from build123d import *

# Parameters (mm, degrees)
BASE_FLANGE1_DEPTH   = 12.5
M4_CLEARANCE_HOLE1_D = 4.5


# Sheet-metal steps are written as plain solids
with BuildPart() as part:
    # Sketch1 → Base-Flange1 (new, symmetric)
    with BuildSketch(Plane(origin=(0, 0, 0), x_dir=(1, 0, 0), z_dir=(0, 1, 0))):
        with BuildLine():
            Line((0, 0), (-12, 0))
            ThreePointArc((-12, 0), (-14.121320344, 0.878679656), (-15, 3))
            Line((-15, 3), (-15, 98.5))
            ThreePointArc((-15, 98.5), (-15.439339828, 99.560660172), (-16.5, 100))
            Line((-16.5, 100), (-95, 100))
            Line((-95, 100), (-95, 101.5))
            Line((-95, 101.5), (-16.5, 101.5))
            ThreePointArc((-16.5, 101.5), (-14.378679656, 100.621320344), (-13.5, 98.5))
            Line((-13.5, 98.5), (-13.5, 3))
            ThreePointArc((-13.5, 3), (-13.060660172, 1.939339828), (-12, 1.5))
            Line((-12, 1.5), (0, 1.5))
            Line((0, 1.5), (0, 0))
        make_face()
    extrude(amount=BASE_FLANGE1_DEPTH, both=True)

    # M4 Clearance Hole1 (through all)
    with Locations(Plane.XY):
        with Locations((-4, 7), (-4, -7)):
            Hole(M4_CLEARANCE_HOLE1_D / 2)


solid = part.part
For this review, take the finished solid that the model builds, in its own axes (mm). A direction names the side the tool comes from. Coordinates: 2 decimals unless noted, no trailing zeros. Loops run counter-clockwise (first coordinate to the right, second up) from the corner with the lowest first, then second, coordinate; pieces in that order, holes last. Notation, with made-up numbers: (-26, 32.25) - (14, 32.25) arc R10 cw to (14, 43.25) - close; hole circle Ø4 at (8.5, -15). An arc over 180 degrees is marked (long way). Use a Markdown table: item, result. Add a question column.
Item 1: Tool access review of faces 5 (the face through (-55, 0, -100)), 6 (the face through (-13.5, 0, -51)), 7 (the face through (-56, 0, -101.5)): name each direction out of +Z, -Z, +X, -X, +Y, -Y from which nothing blocks a thin tool from reaching the whole face with its end or side.
Item 2: Mouldability with a two-part tool opening along X and no side actions: class faces 1 (the face through (-5.21, 8.897, -0.761)), 2 (the face through (-5.21, -5.103, -0.761)), 3 (the face through (-14.1, 0.18, -0.86)), 4 (the face through (-14.4, 0.18, -100.64)) as pulls with the +X half, pulls with the -X half, needs draft (parallel to the pull), parting line crosses it, or undercut.
Item 3: For line 1 (Y direction, x = -4, z = -0.5); line 2 (Z direction, x = -86.5, y = -5); line 3 (X direction, y = -0.75, z = -44), list the stretches that pass through material, from the lowest coordinate up.
Item 4: We need section D-D (x = -49.5). Give the boundary of the cut face in (y, z).
Item 5: We need section B-B (y = 7). Give the boundary of the cut face in (x, z), and give its area (3 significant figures).
Item 6: We need section C-C (z = -77.5). Give the boundary of the cut face in (x, y).
Item 7: Insertion check: pin 1 Ø8 at (y, z) = (-6, -76.5) entering from -X; pin 2 Ø7.5 at (y, z) = (0.5, -30) entering from +X; pin 3 Ø3 at (x, y) = (-29.5, 6) entering from +Z; pin 4 Ø3.5 at (x, y) = (-4, 7) entering from -Z. Each pin has a flat end and moves straight along its axis. Give the tip position at first contact, or say it passes through.
Item 8: We need section A-A (x = -4). Give the boundary of the cut face in (y, z).
Results list:
| question | item | result |
|---|---|---|
| 1 | face 5 | +Z, -X, +Y, -Y |
| 1 | face 6 | -Z, +X, +Y, -Y |
| 1 | face 7 | -Z, +X, -X, +Y, -Y |
| 2 | face 1 | undercut |
| 2 | face 2 | undercut |
| 2 | face 3 | pulls with the -X half |
| 2 | face 4 | pulls with the +X half |
| 3 | line 1 | y = -12.5 to -9.25, -4.75 to 4.75, 9.25 to 12.5 |
| 3 | line 2 | z = -101.5 to -100 |
| 3 | line 3 | x = -15 to -13.5 |
| 4 | outline | (-12.5, -101.5) - (12.5, -101.5) - (12.5, -100) - (-12.5, -100) - close |
| 5 | outline | (-95, -101.5) - (-16.5, -101.5) arc R3 ccw to (-13.5, -98.5) - (-13.5, -3) arc R1.5 cw to (-12, -1.5) - (-6.25, -1.5) - (-6.25, 0) - (-12, 0) arc R3 ccw to (-15, -3) - (-15, -98.5) arc R1.5 cw to (-16.5, -100) - (-95, -100) - close; (-1.75, -1.5) - (0, -1.5) - (0, 0) - (-1.75, 0) - close |
| 5 | area | 283 mm^2 |
| 6 | outline | (-15, -12.5) - (-13.5, -12.5) - (-13.5, 12.5) - (-15, 12.5) - close |
| 7 | pin 1 | stops at x = -15 |
| 7 | pin 2 | stops at x = -13.5 |
| 7 | pin 3 | stops at z = -100 |
| 7 | pin 4 | passes through |
| 8 | outline | (-12.5, -1.5) - (-9.25, -1.5) - (-9.25, 0) - (-12.5, 0) - close; (-4.75, -1.5) - (4.75, -1.5) - (4.75, 0) - (-4.75, 0) - close; (9.25, -1.5) - (12.5, -1.5) - (12.5, 0) - (9.25, 0) - close |
